Design review of the part shown in the three views and the two pictorial views. Dimensions are in mm from the part's minimum x, y and z. Coordinates: 2 decimals unless noted, no trailing zeros. Loops run counter-clockwise (first coordinate to the right, second up) from the corner with the lowest first, then second, coordinate; pieces in that order, holes last. Notation, with made-up numbers: (66.5, 62.25) - (91.5, 62.25) arc R31 ccw to (91.5, 96.25) - close; hole circle Ø6 at (14, 58.25). An arc over 180 degrees is marked (long way). One line per item, written item: value. Start each with the question number.
1. To check wall thickness, follow line 1 (X direction, y = 3.5, z = 2.1); line 2 (X direction, y = 4.5, z = 2.1); line 3 (Y direction, x = 1.5, z = 0.65) (1 decimal). State the ranges of each line that lie inside material, in increasing order. Write a range as from..to.
2. Insertion check: pin 1 (1 mm diameter, centred on x = 1, z = 2, fed in from -Y). The pin has a flat end and moves straight along its axis. Give the tip position at first contact, or say it passes through.
3. Take a section at A-A, the plane z = 0.8. State the section outline as (x, y) points.
4. The part is to be moulded in two halves that separate along X. For the marked faces 1, 2 and 3, say which applies: released by +X, released by -X, zero draft, split by the parting line, or undercut.
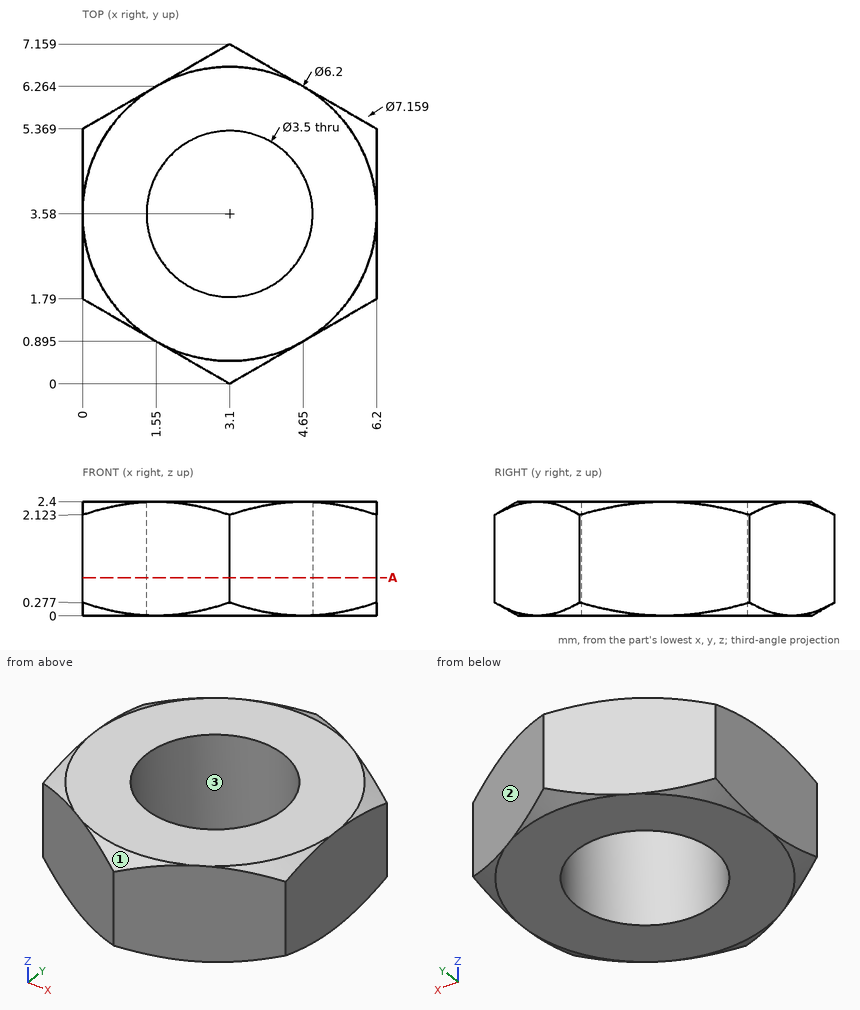
Solutions:
1. line 1: 0..1.35, 4.85..6.2
1. line 2: 0..1.61, 4.59..6.2
1. line 3: 0.9..2.9, 4.3..6.2
2. pin 1: y = 0.92
3. outline: (0, 1.79) - (3.1, 0) - (6.2, 1.79) - (6.2, 5.37) - (3.1, 7.16) - (0, 5.37) - close; hole circle Ø3.5 at (3.1, 3.58)
4. face 1: split by the parting line
4. face 2: released by +X
4. face 3: undercut
